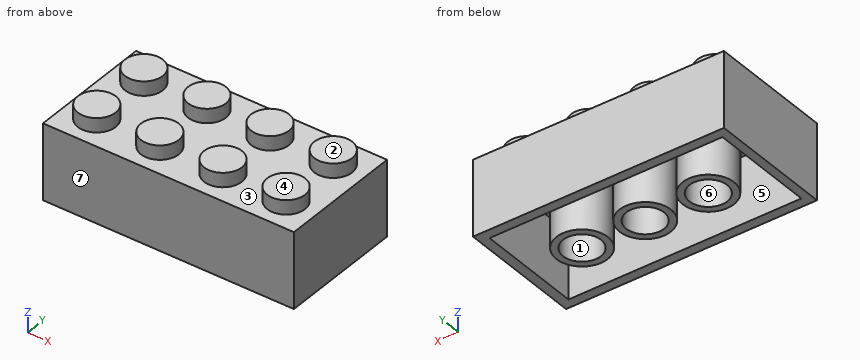
```python
from build123d import *

# Parameters (mm, degrees)
F0_W     = 807.72
F0_H     = 401.32
F1_DEPTH = 243.84
F2_R     = 60.96
F3_DEPTH = 45.72
F4_W     = 749.806969
F4_H     = 340.36
F4_R     = 82.55
F4_R_2   = 60.96
F5_DEPTH = 213.36


with BuildPart() as f1:
    # F0 (on Top) → F1 (new body)
    with BuildSketch(Plane.XY):
        with Locations((-5.254116, 7.858066)):
            Rectangle(F0_W, F0_H)
    extrude(amount=F1_DEPTH)

    # F2 (on face) → F3 (join)
    with BuildSketch(Plane.XY.offset(243.84)):
        with Locations((-310.054116, 109.458066)):
            Circle(F2_R)
        with Locations((-310.054116, -93.741934)):
            Circle(F2_R)
        with Locations((-106.854116, 109.458066)):
            Circle(F2_R)
        with Locations((-106.854116, -93.741934)):
            Circle(F2_R)
        with Locations((96.345884, 109.458066)):
            Circle(F2_R)
        with Locations((96.345884, -93.741934)):
            Circle(F2_R)
        with Locations((299.545884, 109.458066)):
            Circle(F2_R)
        with Locations((299.545884, -93.741934)):
            Circle(F2_R)
    extrude(amount=F3_DEPTH)

    # F4 (on face) → F5 (cut)
    with BuildSketch(Plane(origin=(0, 0, 0), x_dir=(1, 0, 0), z_dir=(0, 0, -1))):
        with Locations((-6.777601, -7.858066)):
            Rectangle(F4_W, F4_H)
        with Locations((-203.2, 0)):
            Circle(F4_R, mode=Mode.SUBTRACT)
        Circle(F4_R, mode=Mode.SUBTRACT)
        with Locations((203.2, 0)):
            Circle(F4_R, mode=Mode.SUBTRACT)
        with Locations((-203.2, 0)):
            Circle(F4_R_2)
        Circle(F4_R_2)
        with Locations((203.2, 0)):
            Circle(F4_R_2)
    extrude(amount=-F5_DEPTH, mode=Mode.SUBTRACT)


solid = f1.part
```
CAD build for the part. Positions are in the model's coordinates, mm. Face numbers are marked on the shaded views. A direction names the side the tool comes from. Coordinates: 2 decimals unless noted, no trailing zeros. Order: outer loops, then holes, each group sorted by start corner. A loop starts at its lowest first (then second) coordinate and runs counter-clockwise, first axis right, second up. Notation, with made-up numbers: M 70.5,-33.5 L 129.5,-33.5 A7 cw 129.5,-24.5 Z; hole C -26.75,-31 d8. An arc over 180 degrees is marked long. Write each question's results on one line, items separated by ' | '. Start each with the question number.
Q1. Cut at D-D (x = -360). List the corners of the cut face in (y, z).
Q2. Cut at B-B (x = -203.2). List the corners of the cut face in (y, z).
Q3. Cut at A-A (z = 72). List the corners of the cut face in (x, y).
Q4. Which spindle directions (+Z, -Z, +X, -X, +Y, -Y) get a long thin tool onto all of the face, cutting with end or side? Do the marked faces 1, 2 and 3. Say none if no direction does.
Q5. Flat gauge pins, fed straight in: P1, Ø5, axis at x = 103.5, y = 104.5, coming from the -Z side; P2, Ø1.5, axis at x = 88, y = 19, coming from the +Z side; P3, Ø12, axis at x = -200.5, z = 255.5, coming from the +Y side. Where does each tip first touch, or does it go through?
Q6. Pull direction Y, two halves, no side cores. Call the marked faces 4, 5, 6 and 7: +Y half, -Y half, draft (parallel to the pull), parting line (faces both ways), or undercut.
Q7. Drill centre lines: probe 1 along Y at (x, z) = (203.2, 67.5); probe 2 along Y at (x, z) = (-205, 85.5); probe 3 along X at (y, z) = (-113, 76.5). Where is each one in solid material? Low to high. Write a range as from..to.
Found:
1) outline: M -192.8,0 L -162.32,0 L -162.32,213.36 L 178.04,213.36 L 178.04,0 L 208.52,0 L 208.52,243.84 L 144.41,243.84 L 144.41,289.56 L 74.51,289.56 L 74.51,243.84 L -58.79,243.84 L -58.79,289.56 L -128.69,289.56 L -128.69,243.84 L -192.8,243.84 Z
2) outline: M -192.8,0 L -162.32,0 L -162.32,213.36 L -82.55,213.36 L -82.55,0 L -60.96,0 L -60.96,213.36 L 60.96,213.36 L 60.96,0 L 82.55,0 L 82.55,213.36 L 178.04,213.36 L 178.04,0 L 208.52,0 L 208.52,243.84 L -192.8,243.84 Z
3) outline: M -409.11,-192.8 L 398.61,-192.8 L 398.61,208.52 L -409.11,208.52 Z; C -203.2,0 d165.1; C 0,0 d165.1; C 203.2,0 d165.1; hole M -381.68,-162.32 L 368.13,-162.32 L 368.13,178.04 L -381.68,178.04 Z; hole C -203.2,0 d121.92; hole C 0,0 d121.92; hole C 203.2,0 d121.92
4) face 1: -Z | face 2: +Z, +X, -X, +Y, -Y | face 3: +Z
5) P1: z = 213.36 | P2: z = 243.84 | P3: through
6) face 4: draft | face 5: undercut | face 6: undercut | face 7: -Y half
7) probe 1: -192.8..-162.32, -82.55..-60.96, 60.96..82.55, 178.04..208.52 | probe 2: -192.8..-162.32, -82.53..-60.93, 60.93..82.53, 178.04..208.52 | probe 3: -409.11..-381.68, 368.13..398.61
